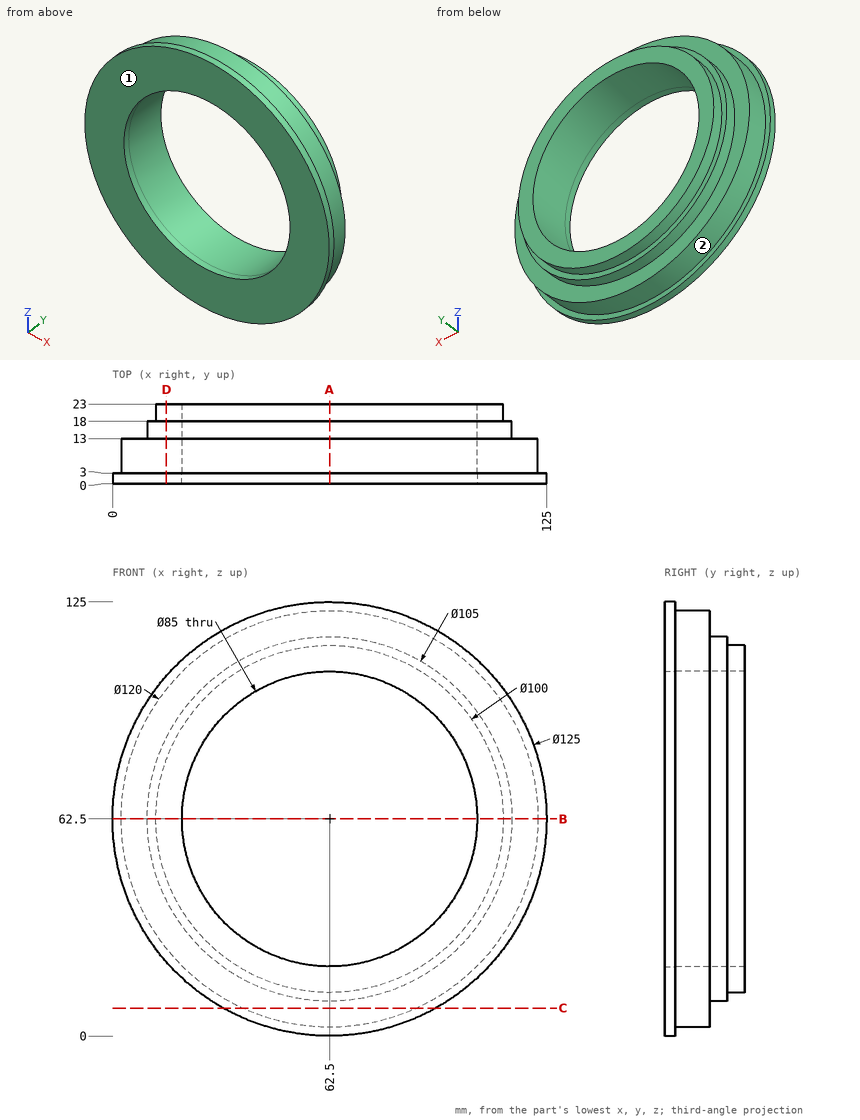
Part print with two shaded views. Sizes in mm from the minimum x, y, z corner. A direction names the side the tool comes from. Coordinates: 2 decimals unless noted, no trailing zeros. Order: outer loops, then holes, each group sorted by start corner. A loop starts at its lowest first (then second) coordinate and runs counter-clockwise, first axis right, second up.
(1) Saw through at C-C, the plane z = 8. Write the cut outline in (x, y), and give its area (3 significant figures).
Solution:
outline: (31.91, 0) - (93.09, 0) - (93.09, 3) - (87.59, 3) - (87.59, 13) - (37.41, 13) - (37.41, 3) - (31.91, 3) - close
area: 685 mm2
(2) Saw through at A-A, the plane x = 62.5. Write the cut outline in (y, z).
Solution:
outline: (0, 0) - (3, 0) - (3, 2.5) - (13, 2.5) - (13, 10) - (18, 10) - (18, 12.5) - (23, 12.5) - (23, 20) - (0, 20) - close; (0, 105) - (23, 105) - (23, 112.5) - (18, 112.5) - (18, 115) - (13, 115) - (13, 122.5) - (3, 122.5) - (3, 125) - (0, 125) - close
(3) Drill centre lines: L1, parallel to Z at x = 62.5, y = 2.45; L2, parallel to X at y = 16, z = 62.5; L3, parallel to X at y = 18.75, z = 62.5. Where is each one in solid material? Low to high.
Solution:
L1: z = 0 to 20, 105 to 125
L2: x = 10 to 20, 105 to 115
L3: x = 12.5 to 20, 105 to 112.5
(4) Saw through at D-D, the plane x = 15.5. Write the cut outline in (y, z).
Solution:
outline: (0, 21.3) - (3, 21.3) - (3, 25.2) - (13, 25.2) - (13, 39.11) - (18, 39.11) - (18, 45.44) - (23, 45.44) - (23, 79.56) - (18, 79.56) - (18, 85.89) - (13, 85.89) - (13, 99.8) - (3, 99.8) - (3, 103.7) - (0, 103.7) - close
(5) Pin check, flat tips, straight feed: pin 1 Ø1.5 at (y, z) = (10, 75) entering from +X; pin 2 Ø4 at (x, y) = (92, 9) entering from +Z; pin 3 Ø8 at (x, y) = (105.5, 19.5) entering from -Z. Stop position of each tip, or through.
Solution:
pin 1: stops at x = 121.34
pin 2: stops at z = 115.83
pin 3: stops at z = 27.68
(6) Which spindle directions (+Z, -Z, +X, -X, +Y, -Y) get a long thin tool onto all of the face, cutting with end or side? Do the marked faces 1 and 2. Say none if no direction does.
Solution:
face 1: +Z, -Z, +X, -X, -Y
face 2: +Y
(7) Saw through at B-B, the plane z = 62.5. Write the cut outline in (x, y).
Solution:
outline: (0, 0) - (20, 0) - (20, 23) - (12.5, 23) - (12.5, 18) - (10, 18) - (10, 13) - (2.5, 13) - (2.5, 3) - (0, 3) - close; (105, 0) - (125, 0) - (125, 3) - (122.5, 3) - (122.5, 13) - (115, 13) - (115, 18) - (112.5, 18) - (112.5, 23) - (105, 23) - close
